Verification items for the finished model (mm, model axes). A direction names the side the tool comes from. Round coordinates to 2 decimals unless told otherwise and drop trailing zeros. Loops run counter-clockwise (first coordinate to the right, second up) from the corner with the lowest first, then second, coordinate; pieces in that order, holes last. Notation, with made-up numbers: (-15, 12) - (-2, 12) arc R29 cw to (-2, 41) - close; hole circle Ø8 at (0.25, -5.5). An arc over 180 degrees is marked (long way). Use CSV: the item, a comma, the result in double quotes.
```python
from build123d import *

# Parameters (mm, degrees)
PAD001_DEPTH  = 10.5
SKETCH002_R   = 5.35
SKETCH002_R_2 = 3.175
PAD002_DEPTH  = 8.5
SKETCH003_R   = 4.5
PAD003_DEPTH  = 3.7
CHAMFER_SIZE  = 1
SKETCH006_W   = 4
SKETCH006_H   = 4
PAD005_DEPTH  = 6
FILLET_R      = 1


with BuildPart() as part:
    # Sketch001 → Pad001 (new body, symmetric)
    with BuildSketch(Plane.YZ):
        with BuildLine():
            Line((8, 17.35), (8, 20))
            Line((8, 20), (0, 20))
            Line((0, 20), (0, 0))
            Line((0, 0), (8, 0))
            Line((8, 2.65), (8, 0))
            ThreePointArc((8, 2.65), (15.35, 10), (8, 17.35))
        make_face()
    extrude(amount=PAD001_DEPTH, both=True)

    # Sketch002 (on Face8 of Pad001) → Pad002 (join)
    with BuildSketch(Plane.YZ.offset(10.5)):
        with Locations((8, 10)):
            Circle(SKETCH002_R)
        with Locations((8, 10)):
            Circle(SKETCH002_R_2, mode=Mode.SUBTRACT)
    extrude(amount=PAD002_DEPTH)

    # Sketch003 (on Face4 of Pad002) → Pad003 (join)
    with BuildSketch(Plane(origin=(-10.5, 0, 0), x_dir=(0, 1, 0), z_dir=(-1, 0, 0))):
        with Locations((8, -10)):
            Circle(SKETCH003_R)
    extrude(amount=PAD003_DEPTH)

    # Chamfer
    chamfer_edges = [part.edges().sort_by_distance(p)[0] for p in [
        (-14.2, 3.5, 10),
        (19, 2.65, 10),
    ]]
    chamfer(chamfer_edges, length=CHAMFER_SIZE)

    # Sketch006 (on Face6 of Chamfer) → Pad005 (join)
    with BuildSketch(Plane.ZX.offset(8)):
        with Locations((2.5, -6.5)):
            Rectangle(SKETCH006_W, SKETCH006_H)
        with Locations((2.5, 6.5)):
            Rectangle(SKETCH006_W, SKETCH006_H)
    extrude(amount=PAD005_DEPTH)

    # Fillet
    fillet_edges = [part.edges().sort_by_distance(p)[0] for p in [
        (-6.5, 14, 0.5),
        (6.5, 14, 0.5),
        (-6.5, 14, 4.5),
        (6.5, 14, 4.5),
    ]]
    fillet(fillet_edges, radius=FILLET_R)


solid = part.part
```
1) Mould release check, pull along Z, two halves, no side actions. Record for faces 5 (the face through (0, 0, 10)), 6 (the face through (6, 10, 0.5)), 7 (the face through (-6.472, 13.715, 4.199)): +Z half, -Z half, draft (parallel to the pull), parting line (faces both ways), or undercut.
Returned:
face 5,"draft"
face 6,"-Z half"
face 7,"undercut"
2) Cross-section at D-D, the plane y = 1.25. Record the cut outline in (x, z).
Returned:
outline,"(-10.5, 0) - (10.5, 0) - (10.5, 20) - (-10.5, 20) - close"
3) Cross-section at C-C, the plane x = 14.5. Record the cut outline in (y, z) (3 decimals).
Returned:
outline,"circle Ø10.7 at (8, 10); hole circle Ø6.35 at (8, 10)"
4) Cross-section at B-B, the plane x = -1. Record the cut outline in (y, z).
Returned:
outline,"(0, 0) - (8, 0) - (8, 2.65) arc R7.35 ccw to (8, 17.35) - (8, 20) - (0, 20) - close"
5) Gauge pin test, flat ends, axial feed: pin 1 Ø6 at (y, z) = (4.5, 4) entering from +X; pin 2 Ø3 at (x, y) = (-5.5, 10) entering from -Z; pin 3 Ø3 at (y, z) = (10, 2) entering from +X; pin 4 Ø1.3 at (x, z) = (-4.5, 19) entering from +Y. Record the tip position at first contact, or that the pin passes through.
Returned:
pin 1,"stops at x = 19"
pin 2,"stops at z = 0.5"
pin 3,"stops at x = 10.5"
pin 4,"stops at y = 8"
6) Access from +Z, -Z, +X, -X, +Y, -Y to the whole of each face (thin tool, end or side, straight path). Record for faces 1 (the face through (-6, 14, 2)), 2 (the face through (-8.5, 12, 2)), 3 (the face through (10.5, 8, 10)), 4 (the face through (4.5, 12, 2)).
Returned:
face 1,"-Z, +X, -X, +Y"
face 2,"-Z, -X, +Y"
face 3,"+X"
face 4,"-Z, +Y"
7) Thickness scan on probe 1 along Z at (x, y) = (13.25, 8) (3 decimals); probe 2 along X at (y, z) = (12, 1.5); probe 3 along X at (y, z) = (10.5, 15.75). Record the ranges inside material, lowest first. Write a range as [from, to].
Returned:
probe 1,"z = [4.65, 6.825], [13.175, 15.35]"
probe 2,"x = [-8.5, -4.5], [4.5, 8.5]"
probe 3,"x = [-10.5, 10.5]"
8) Cross-section at A-A, the plane z = 10. Record the cut outline in (x, y) (3 decimals), then the cut area to 3 significant figures.
Returned:
outline,"(-14.2, 4.5) - (-13.2, 3.5) - (-10.5, 3.5) - (-10.5, 0) - (10.5, 0) - (10.5, 2.65) - (18, 2.65) - (19, 3.65) - (19, 4.825) - (10.5, 4.825) - (10.5, 11.175) - (19, 11.175) - (19, 12.35) - (18, 13.35) - (10.5, 13.35) - (10.5, 15.35) - (-10.5, 15.35) - (-10.5, 12.5) - (-13.2, 12.5) - (-14.2, 11.5) - close"
area,"391 mm²"
